from build123d import *

# Parameters (mm, degrees)
BOSS_EXTRUDE1_DEPTH                            = 4.7625
SKETCH4_W                                      = 6.604
SKETCH4_H                                      = 2.54
BOSS_EXTRUDE2_DEPTH                            = 6.35
CBORE_FOR_6_BUTTON_HEAD_CAP_SCREW1_D           = 3.6576
CBORE_FOR_6_BUTTON_HEAD_CAP_SCREW1_DEPTH       = 6.35
CBORE_FOR_6_BUTTON_HEAD_CAP_SCREW1_CBORE_D     = 7.54126
CBORE_FOR_6_BUTTON_HEAD_CAP_SCREW1_CBORE_DEPTH = 1.8542


with BuildPart() as part:
    # Sketch1 → Boss-Extrude1 (new, symmetric)
    with BuildSketch(Plane.XY):
        with BuildLine():
            Line((6.52733268, -50.8), (0, -36.802089895))
            Line((0, -36.802089895), (-6.52733268, -50.8))
            Line((-6.52733268, -50.8), (-19.05, -50.8))
            Line((-19.05, -50.8), (-19.05, -44.45))
            Line((-19.05, -44.45), (-10.16, -44.45))
            add(Edge.make_bspline(
                [(-12.7, -10.045250432), (0.767706839, -28.651479816), (-10.16, -44.45)],
                knots=[0, 0, 0, 1, 1, 1], degree=2))
            ThreePointArc((-12.7, -10.045250432), (-15.29447296, -5.317532616), (-16.1925, 0))
            Line((-16.1925, 0), (-11.43, 0))
            ThreePointArc((-11.43, 0), (0, -11.43), (11.43, 0))
            Line((11.43, 0), (16.1925, 0))
            ThreePointArc((16.1925, 0), (15.29447296, -5.317532616), (12.7, -10.045250432))
            add(Edge.make_bspline(
                [(12.7, -10.045250432), (-0.767706839, -28.651479816), (10.16, -44.45)],
                knots=[0, 0, 0, 1, 1, 1], degree=2))
            Line((10.16, -44.45), (19.05, -44.45))
            Line((19.05, -44.45), (19.05, -50.8))
            Line((19.05, -50.8), (6.52733268, -50.8))
        make_face()
        Polygon((4.254975404, -16.1925), (-4.254975404, -16.1925), (0, -27.277089895), align=None, mode=Mode.SUBTRACT)
    extrude(amount=BOSS_EXTRUDE1_DEPTH, both=True)

    # Sketch4 → Cut-Revolve1 (revolve, cut)
    with BuildSketch(Plane(origin=(0, 0, 0), x_dir=(0, 0, -1), z_dir=(1, 0, 0))):
        with Locations((0, -12.7)):
            Rectangle(SKETCH4_W, SKETCH4_H)
    revolve(axis=Axis((0, 0, 0), (0, 0, -1)), mode=Mode.SUBTRACT)

    # Sketch8 → Boss-Extrude2 (add)
    with BuildSketch(Plane(origin=(0, -44.45, 0), x_dir=(1, 0, 0), z_dir=(0, 1, 0))):
        with BuildLine():
            Line((-19.05, 4.7625), (-19.05, -4.7625))
            ThreePointArc((-19.05, -4.7625), (-23.8125, 0), (-19.05, 4.7625))
        make_face()
        with BuildLine():
            Line((19.05, 4.7625), (19.05, -4.7625))
            ThreePointArc((19.05, -4.7625), (23.8125, 0), (19.05, 4.7625))
        make_face()
    extrude(amount=-BOSS_EXTRUDE2_DEPTH)

    # CBORE for #6 Button Head Cap Screw1
    with Locations(Plane(origin=(0, -44.45, 0), x_dir=(1, 0, 0), z_dir=(0, 1, 0))):
        with Locations((-19.05, 0), (19.05, 0)):
            CounterBoreHole(CBORE_FOR_6_BUTTON_HEAD_CAP_SCREW1_D / 2, CBORE_FOR_6_BUTTON_HEAD_CAP_SCREW1_CBORE_D / 2, CBORE_FOR_6_BUTTON_HEAD_CAP_SCREW1_CBORE_DEPTH, depth=CBORE_FOR_6_BUTTON_HEAD_CAP_SCREW1_DEPTH)


solid = part.part
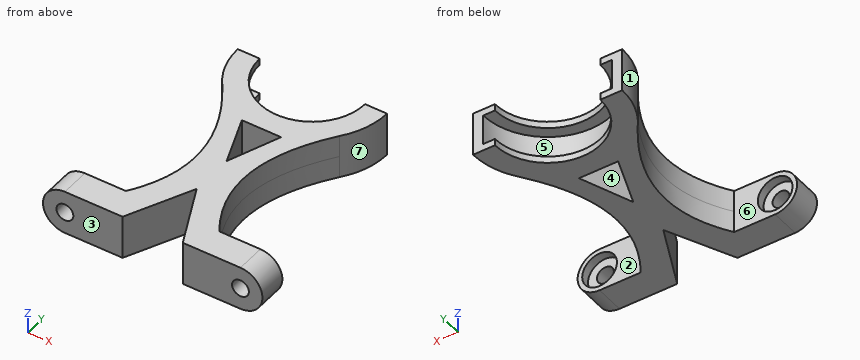
Geometry check sheet. Reference: the model listing, model coordinates, mm. Face numbers are marked on the shaded views. A direction names the side the tool comes from. Coordinates: 2 decimals unless noted, no trailing zeros. Loops run counter-clockwise (first coordinate to the right, second up) from the corner with the lowest first, then second, coordinate; pieces in that order, holes last. Notation, with made-up numbers: (54, -22) - (98, -22) arc R20 ccw to (98, 1) - close; hole circle Ø5 at (-38, -25). An arc over 180 degrees is marked (long way). Use one line per item in the form item = value. Start each with the question number.
Item 1: Section check B-B, the plane z = 1. Give the number of separate pieces and of enclosed holes in the cut face, and give its area (3 significant figures).
Item 2: Tool access check on the marked faces 1, 2, 3 and 4. Record the directions out of +Z, -Z, +X, -X, +Y, -Y that give a thin tool (end or side, any length) a straight path to the whole face; none if there is none.
Item 3: Section check A-A, the plane x = -2.5. Enter the section's corners in (y, z), and give its area (3 significant figures).
Item 4: Thickness scan on probe 1 along Z at (x, y) = (-19, -49); probe 2 along X at (y, z) = (-30, -2.5); probe 3 along Y at (x, z) = (-10, 1.25). Record the ranges inside material, lowest first.
Item 5: Gauge pin test, flat ends, axial feed: pin 1 (4.5 mm diameter, centred on x = 0.5, z = 2, fed in from -Y); pin 2 (2 mm diameter, centred on y = -25.5, z = -3.5, fed in from +X); pin 3 (3.5 mm diameter, centred on x = -19.05, z = 0, fed in from +Y); pin 4 (3 mm diameter, centred on x = -20.5, z = 2, fed in from +Y). Record the tip position at first contact, or that the pin passes through.
Item 6: Mould release check, pull along X, two halves, no side actions. Record for the marked faces 5, 6 and 7: +X half, -X half, draft (parallel to the pull), parting line (faces both ways), or undercut.
Computed:
q1.separate_pieces = 3
q1.enclosed_holes = 1
q1.area = 614 mm2
q2.face_1 = +Z, -Z, -X
q2.face_2 = +Z, -Z, +X
q2.face_3 = +Z, -Z, +X, -X, -Y
q2.face_4 = +Z, -Z
q3.outline = (-42.16, -4.76) - (-20.76, -4.76) - (-20.76, 4.76) - (-42.16, 4.76) - close; (-16.19, -4.76) - (-11.15, -4.76) - (-11.15, -3.3) - (-13.74, -3.3) - (-13.74, 3.3) - (-11.15, 3.3) - (-11.15, 4.76) - (-16.19, 4.76) - close
q3.area = 235 mm2
q4.probe_1 = -4.76 to -1.83, 1.83 to 4.76
q4.probe_2 = -5.27 to 5.27
q4.probe_3 = -50.8 to -44.22, -14.16 to -9.76
q5.pin_1 = -42.7
q5.pin_2 = 5.83
q5.pin_3 = through
q5.pin_4 = -44.45
q6.face_5 = undercut
q6.face_6 = draft
q6.face_7 = +X half
